```python
from build123d import *

# Parameters (mm, degrees)
SKETCH1_W                     = 90
SKETCH1_H                     = 22
BASE_FLANGE1_DEPTH            = 2
EDGE_FLANGE4_STRIP_W          = 10
EDGE_FLANGE4_STRIP_H          = 2
EDGE_FLANGE4_STRIP_CUT_DEPTH  = 32
EDGE_FLANGE4_RELIEF_W         = 11
EDGE_FLANGE4_RELIEF_H         = 1
EDGE_FLANGE4_RELIEF_CUT_DEPTH = 2
EDGE_FLANGE4_DEPTH            = 32
EDGE_FLANGE8_DEPTH            = 16
EDGE_FLANGE9_DEPTH            = 16
FILLET2_R                     = 1
FILLET4_R                     = 1
FILLET5_R                     = 1
FILLET7_R                     = 0.5
FILLET8_R                     = 0.5
FILLET9_R                     = 0.5
FILLET10_R                    = 1
BREAK_CORNER2_START           = -39.597979746
BREAK_CORNER2_OUTLINE_W       = 72.124891682
BREAK_CORNER2_OUTLINE_H       = 4
BREAK_CORNER2_DEPTH           = 3.535533905
BREAK_CORNER2_START_2         = 36.062445841
BREAK_CORNER2_2_OUTLINE_W     = 72.124891682
BREAK_CORNER2_2_OUTLINE_H     = 4
BREAK_CORNER2_2_DEPTH         = 3.535533905
BREAK_CORNER2_START_3         = -27.577164466
BREAK_CORNER2_3_OUTLINE_W     = 3.937554159
BREAK_CORNER2_3_OUTLINE_H     = 4
BREAK_CORNER2_3_DEPTH         = 55.154328932
FILLET11_R                    = 1
FILLET12_R                    = 0.5
FILLET13_R                    = 1
SKETCH62_R                    = 4
CUT_EXTRUDE2_DEPTH            = 10
SKETCH63_R                    = 4
CUT_EXTRUDE3_DEPTH            = 10


# Read off the part's stored shape, not the designer's step: Break-Corner2
# Sheet-metal steps are written as plain solids
with BuildPart() as part:
    # Sketch1 → Base-Flange1 (new body)
    with BuildSketch(Plane(origin=(0, 0, 0), x_dir=(1, 0, 0), z_dir=(0, 1, 0))):
        Rectangle(SKETCH1_W, SKETCH1_H)
    extrude(amount=-BASE_FLANGE1_DEPTH)

    # Edge-Flange4 strip (across the edge) → Edge-Flange4 strip cut (cut)
    with BuildSketch(Plane(origin=(-16, 0, 11), x_dir=(0, 0, -1), z_dir=(1, 0, 0))):
        with Locations((-2, -1)):
            Rectangle(EDGE_FLANGE4_STRIP_W, EDGE_FLANGE4_STRIP_H)
    edge_flange4_strip_cut = extrude(amount=EDGE_FLANGE4_STRIP_CUT_DEPTH, mode=Mode.SUBTRACT)

    # Edge-Flange4 relief (on the sheet) → Edge-Flange4 relief cut (cut)
    with BuildSketch(Plane(origin=(-16, 0, 8), x_dir=(0, 0, -1), z_dir=(0, 1, 0))):
        with Locations((-4.5, 0.5)):
            Rectangle(EDGE_FLANGE4_RELIEF_W, EDGE_FLANGE4_RELIEF_H)
        with Locations((-4.5, -32.5)):
            Rectangle(EDGE_FLANGE4_RELIEF_W, EDGE_FLANGE4_RELIEF_H)
    edge_flange4_relief_cut = extrude(amount=-EDGE_FLANGE4_RELIEF_CUT_DEPTH, mode=Mode.SUBTRACT)

    # Edge-Flange4 section (across the edge) → Edge-Flange4 (add)
    with BuildSketch(Plane(origin=(-16, 0, 11), x_dir=(0, 0, -1), z_dir=(1, 0, 0))):
        with BuildLine():
            Line((0, 1), (0, 18))
            Line((0, 18), (2, 18))
            Line((2, 18), (2, 1))
            ThreePointArc((2, 1), (2.292893219, 0.292893219), (3, 0))
            Line((3, 0), (3, -2))
            ThreePointArc((3, -2), (0.878679656, -1.121320344), (0, 1))
        make_face()
    edge_flange4 = extrude(amount=EDGE_FLANGE4_DEPTH)

    # Edge-Flange8 section (across the edge) → Edge-Flange8 (add)
    with BuildSketch(Plane(origin=(17, 18, 9), x_dir=(-1, 0, 0), z_dir=(0, -1, 0))):
        with BuildLine():
            Line((-2, 1), (-2, 6))
            Line((-2, 6), (0, 6))
            Line((0, 6), (0, 1))
            ThreePointArc((0, 1), (0.292893219, 0.292893219), (1, 0))
            Line((1, 0), (1, -2))
            ThreePointArc((1, -2), (-1.121320344, -1.121320344), (-2, 1))
        make_face()
    edge_flange8 = extrude(amount=EDGE_FLANGE8_DEPTH)

    # Edge-Flange9 section (across the edge) → Edge-Flange9 (add)
    with BuildSketch(Plane(origin=(-17, 2, 9), x_dir=(1, 0, 0), z_dir=(0, 1, 0))):
        with BuildLine():
            Line((-2, 1), (-2, 5))
            Line((-2, 5), (0, 5))
            Line((0, 5), (0, 1))
            ThreePointArc((0, 1), (0.292893219, 0.292893219), (1, 0))
            Line((1, 0), (1, -2))
            ThreePointArc((1, -2), (-1.121320344, -1.121320344), (-2, 1))
        make_face()
    edge_flange9 = extrude(amount=EDGE_FLANGE9_DEPTH)

    # Fillet2
    fillet2_edges = [part.edges().sort_by_distance(p)[0] for p in [
        (18, 2, 3),
    ]]
    fillet(fillet2_edges, radius=FILLET2_R)

    # Fillet4
    fillet4_edges = [part.edges().sort_by_distance(p)[0] for p in [
        (-18, 18, 4),
        (18, 18, 3),
    ]]
    fillet(fillet4_edges, radius=FILLET4_R)

    # Fillet5
    fillet5_edges = [part.edges().sort_by_distance(p)[0] for p in [
        (-18, 2, 4),
    ]]
    fillet(fillet5_edges, radius=FILLET5_R)

    # Fillet7
    fillet7_edges = [part.edges().sort_by_distance(p)[0] for p in [
        (16, -1, 7),
    ]]
    fillet(fillet7_edges, radius=FILLET7_R)

    # Fillet8
    fillet8_edges = [part.edges().sort_by_distance(p)[0] for p in [
        (17, -1, 7),
    ]]
    fillet(fillet8_edges, radius=FILLET8_R - 0.0001)  # a hair under: the kernel refuses the full size

    # Fillet9
    fillet9_edges = [part.edges().sort_by_distance(p)[0] for p in [
        (-16, -1, 7),
        (-17, -1, 7),
    ]]
    fillet(fillet9_edges, radius=FILLET9_R - 0.0001)  # a hair under: the kernel refuses the full size

    # Fillet10
    fillet10_edges = [part.edges().sort_by_distance(p)[0] for p in [
        (17, -1, 11),
        (-17, -1, 11),
    ]]
    fillet(fillet10_edges, radius=FILLET10_R)

    # Break-Corner2 outline → Break-Corner2 (cut)
    with BuildSketch(Plane(origin=(0, 0, 0), x_dir=(0.7071067811865471, 0, -0.707106781186548), z_dir=(0.707106781186548, 0, 0.707106781186547)).offset(BREAK_CORNER2_START)):
        with Locations((0, -1)):
            Rectangle(BREAK_CORNER2_OUTLINE_W, BREAK_CORNER2_OUTLINE_H)
    extrude(amount=BREAK_CORNER2_DEPTH, mode=Mode.SUBTRACT)

    # Break-Corner2 2 outline → Break-Corner2 2 (cut)
    with BuildSketch(Plane(origin=(0, 0, 0), x_dir=(0.7071067811865471, 0, -0.707106781186548), z_dir=(0.707106781186548, 0, 0.707106781186547)).offset(BREAK_CORNER2_START_2)):
        with Locations((0, -1)):
            Rectangle(BREAK_CORNER2_2_OUTLINE_W, BREAK_CORNER2_2_OUTLINE_H)
    extrude(amount=BREAK_CORNER2_2_DEPTH, mode=Mode.SUBTRACT)

    # Break-Corner2 3 outline → Break-Corner2 3 (cut)
    with BuildSketch(Plane(origin=(0, 0, 0), x_dir=(0.7071067811865471, 0, -0.707106781186548), z_dir=(0.707106781186548, 0, 0.707106781186547)).offset(BREAK_CORNER2_START_3)):
        with Locations((38.03122292, -1)):
            Rectangle(BREAK_CORNER2_3_OUTLINE_W, BREAK_CORNER2_3_OUTLINE_H)
        with Locations((-38.03122292, -1)):
            Rectangle(BREAK_CORNER2_3_OUTLINE_W, BREAK_CORNER2_3_OUTLINE_H)
    extrude(amount=BREAK_CORNER2_3_DEPTH, mode=Mode.SUBTRACT)

    # Mirror1: Edge-Flange4 strip cut, Edge-Flange4 relief cut, Edge-Flange4, Edge-Flange8, Edge-Flange9 across plane
    add(edge_flange4_strip_cut.mirror(Plane.XY), mode=Mode.SUBTRACT)
    add(edge_flange4_relief_cut.mirror(Plane.XY), mode=Mode.SUBTRACT)
    add(edge_flange4.mirror(Plane.XY))
    add(edge_flange8.mirror(Plane.XY))
    add(edge_flange9.mirror(Plane.XY))

    # Fillet11
    fillet11_edges = [part.edges().sort_by_distance(p)[0] for p in [
        (17, -1, -11),
        (-17, -1, -11),
        (-18, 2, -4),
        (-18, 18, -4),
        (18, 2, -3),
        (18, 18, -3),
    ]]
    fillet(fillet11_edges, radius=FILLET11_R)

    # Fillet12
    fillet12_edges = [part.edges().sort_by_distance(p)[0] for p in [
        (-17, -1, -7),
        (-16, -1, -7),
        (16, -1, -7),
        (17, -1, -7),
    ]]
    fillet(fillet12_edges, radius=FILLET12_R - 0.0001)  # a hair under: the kernel refuses the full size

    # Fillet13
    fillet13_edges = [part.edges().sort_by_distance(p)[0] for p in [
        (40.000000001, -1, 11),
        (45, -1, 6.000000001),
        (45, -1, -6.000000001),
        (40.000000001, -1, -11),
        (-40.000000001, -1, -11),
        (-45, -1, -6.000000001),
        (-45, -1, 6.000000001),
        (-40.000000001, -1, 11),
    ]]
    fillet(fillet13_edges, radius=FILLET13_R)

    # Sketch62 → Cut-Extrude2 (cut)
    with BuildSketch(Plane(origin=(0, 0, 0), x_dir=(1, 0, 0), z_dir=(0, 1, 0))):
        with Locations(Location((-32, 0, 0), (0, 0, 270))):
            Circle(SKETCH62_R)
    extrude(amount=-CUT_EXTRUDE2_DEPTH, mode=Mode.SUBTRACT)

    # Sketch63 → Cut-Extrude3 (cut)
    with BuildSketch(Plane(origin=(0, 0, 0), x_dir=(1, 0, 0), z_dir=(0, 1, 0))):
        with Locations(Location((32, 0, 0), (0, 0, 270))):
            Circle(SKETCH63_R)
    extrude(amount=-CUT_EXTRUDE3_DEPTH, mode=Mode.SUBTRACT)


solid = part.part
```
The model under review builds one solid part; all positions refer to its coordinate system, in mm. A direction names the side the tool comes from. Coordinates: 2 decimals unless noted, no trailing zeros. Write each loop counter-clockwise with the first axis right and the second up, starting at its lowest first coordinate (ties: lowest second). Pieces come first, ordered by that corner, then holes. Notation, with made-up numbers: (89.5, 79) -> (122.5, 79) arc R17 cw to (122.5, 86) -> close; hole circle Ø8 at (66, 32.5). An arc over 180 degrees is marked (long way). One line per item, written item: value. Start each with the question number.
Q1. The part is to be moulded in two halves that separate along X. For faces 1 (the face through (-45, -1, 0)), 2 (the face through (35.966, -0.986, -0.521)), 3 (the face through (42, -1, 9)), say which applies: +X half, -X half, draft (parallel to the pull), parting line (faces both ways), or undercut.
Q2. Add section B-B, the plane z = -2. Give the boundary of the cut face in (x, y).
Q3. Clearance check with flat-ended pins moving along their axes: P1, Ø2, axis at y = 8.5, z = -6.5, coming from the -X side; P2, Ø0.6, axis at y = -1, z = -8.5, coming from the -X side; P3, Ø3, axis at y = 0, z = -9.5, coming from the +X side. State where each tip first meets the part, or that it passes through.
Q4. Add section D-D, the plane x = 8. Give the boundary of the cut face in (y, z).
Q5. Add section A-A, the plane x = 32. Give the boundary of the cut face in (y, z), then the cut area to 3 significant figures.
Q6. Add section C-C, the plane y = 11.25. Give the boundary of the cut face in (x, z).
Q7. To check wall thickness, follow probe 1 along X at (y, z) = (-0.55, 0); probe 2 along Z at (x, y) = (13.5, 17.25); probe 3 along Y at (x, z) = (-17.5, 7). State the ranges of each line that lie inside material, in increasing order.
Q8. For faces 4 (the face through (18, 10, 3)), 5 (the face through (19, 10, 6)), 6 (the face through (-16, 0, -9)), list the 3-axis set-ups (+Z, -Z, +X, -X, +Y, -Y) from which the entire face can be reached by the end or side of a thin tool; tool diameter is ignored.
Response:
1. face 1: -X half
1. face 2: undercut
1. face 3: +X half
2. outline: (-45, -2) -> (-35.46, -2) -> (-35.46, 0) -> (-45, 0) -> close; (-28.54, -2) -> (28.54, -2) -> (28.54, 0) -> (-28.54, 0) -> close; (35.46, -2) -> (45, -2) -> (45, 0) -> (35.46, 0) -> close
3. P1: x = -19
3. P2: x = -42.8
3. P3: x = 43
4. outline: (-2, -8) arc R3 ccw to (1, -11) -> (18, -11) -> (18, -9) -> (1, -9) arc R1 cw to (0, -8) -> (0, 8) arc R1 cw to (1, 9) -> (18, 9) -> (18, 11) -> (1, 11) arc R3 ccw to (-2, 8) -> close
5. outline: (-2, -11) -> (0, -11) -> (0, -4) -> (-2, -4) -> close; (-2, 4) -> (0, 4) -> (0, 11) -> (-2, 11) -> close
5. area: 28.0 mm²
6. outline: (-19, -8) arc R3 ccw to (-16, -11) -> (16, -11) arc R3 ccw to (19, -8) -> (19, -3) -> (17, -3) -> (17, -8) arc R1 cw to (16, -9) -> (-16, -9) arc R1 cw to (-17, -8) -> (-17, -4) -> (-19, -4) -> close; (-19, 4) -> (-17, 4) -> (-17, 8) arc R1 cw to (-16, 9) -> (16, 9) arc R1 cw to (17, 8) -> (17, 3) -> (19, 3) -> (19, 8) arc R3 ccw to (16, 11) -> (-16, 11) arc R3 ccw to (-19, 8) -> close
7. probe 1: -45 to -36, -28 to 28, 36 to 45
7. probe 2: -11 to -9, 9 to 11
7. probe 3: -2 to 0, 2 to 18
8. face 4: +X, -X, +Y
8. face 5: +Z, -Z, +X, +Y
8. face 6: -Z, -Y
